Model file for the job. Use its own axes, mm. A direction names the side the tool comes from. Coordinates: 2 decimals unless noted, no trailing zeros. Loops run counter-clockwise (first coordinate to the right, second up) from the corner with the lowest first, then second, coordinate; pieces in that order, holes last. Notation, with made-up numbers: M -30.5,-29.5 L 8.5,-29.5 A16 ccw 8.5,-2.5 Z; hole C 43.5,59.25 d7. An arc over 180 degrees is marked long. One line per question, with ' | ' between items. Start each with the question number.
```python
from build123d import *

# Parameters (mm, degrees)
PAD_DEPTH       = 99.5
POCKET_DEPTH    = 106.001
POCKET001_DEPTH = 105
POCKET002_DEPTH = 37
POCKET003_DEPTH = 37
SKETCH005_W     = 30
SKETCH005_H     = 16.444138
POCKET004_DEPTH = 149


with BuildPart() as part:
    # Sketch → Pad (new body)
    with BuildSketch(Plane.XY):
        with BuildLine():
            Line((-53, 15), (-53, -29))
            ThreePointArc((-53, -29), (0, -82), (53, -29))
            Line((53, 15), (53, -29))
            ThreePointArc((53, 15), (48.606602, 25.606602), (38, 30))
            Line((-38, 30), (38, 30))
            ThreePointArc((-38, 30), (-48.606602, 25.606602), (-53, 15))
        make_face()
    extrude(amount=PAD_DEPTH)

    # Sketch001 (on DatumPlane) → Pocket (cut, through all)
    with BuildSketch(Plane.YZ.offset(53)):
        with BuildLine():
            ThreePointArc((30, 99.5), (-33.496233, 81.683249), (-82, 37))
            Line((-82, 37), (-89.555687, 37))
            Line((-89.555687, 106.401093), (-89.555687, 37))
            Line((30, 106.401093), (-89.555687, 106.401093))
            Line((30, 99.5), (30, 106.401093))
        make_face()
    extrude(amount=-POCKET_DEPTH, mode=Mode.SUBTRACT)

    # Sketch002 (on DatumPlane) → Pocket001 (cut)
    with BuildSketch(Plane.XY.offset(106)):
        with BuildLine():
            Line((-52, -29), (-16, -29))
            Line((-16, -29), (-16, -78.477268))
            ThreePointArc((-52, -29), (-42.047592, -59.594117), (-16, -78.477268))
        make_face()
        with BuildLine():
            Line((-15, 29), (15, 29))
            Line((15, 29), (15, -78.789557))
            ThreePointArc((-15, -78.789557), (0, -81), (15, -78.789557))
            Line((-15, 29), (-15, -78.789557))
        make_face()
        with BuildLine():
            Line((52, -29), (16, -29))
            Line((16, -29), (16, -78.477268))
            ThreePointArc((16, -78.477268), (42.047592, -59.594117), (52, -29))
        make_face()
        with BuildLine():
            Line((-16, 29), (-38.000001, 29))
            ThreePointArc((-38.000001, 29), (-47.850607, 24.850607), (-52, 15))
            Line((-52, 15), (-52, -28))
            Line((-52, -28), (-16, -28))
            Line((-16, -28), (-16, 29))
        make_face()
        with BuildLine():
            Line((16, 29), (38, 29))
            ThreePointArc((52, 15), (47.899495, 24.899495), (38, 29))
            Line((52, 15), (52, -28))
            Line((52, -28), (16, -28))
            Line((16, -28), (16, 29))
        make_face()
    extrude(amount=-POCKET001_DEPTH, mode=Mode.SUBTRACT)

    # Sketch003 (on DatumPlane) → Pocket002 (cut)
    with BuildSketch(Plane.YZ.offset(53)):
        Polygon((-29, 19), (-81, 19), (-81, 99.5), (-29.5, 99.5), (30, 99.5), (30, 82), (-29, 82), align=None)
    extrude(amount=-POCKET002_DEPTH, mode=Mode.SUBTRACT)

    # Sketch004 (on DatumPlane) → Pocket003 (cut)
    with BuildSketch(Plane(origin=(-53, 0, 0), x_dir=(0, -1, 0), z_dir=(-1, 0, 0))):
        Polygon((81, 38), (29, 38), (29, 68), (-30, 68), (-30, 99.5), (81, 99.5), align=None)
    extrude(amount=-POCKET003_DEPTH, mode=Mode.SUBTRACT)

    # Sketch005 (on DatumPlane) → Pocket004 (cut)
    with BuildSketch(Plane(origin=(-53, -120, 0), x_dir=(1, 0, 0), z_dir=(0, -1, 0))):
        with Locations((53, 46.222069)):
            Rectangle(SKETCH005_W, SKETCH005_H)
    extrude(amount=-POCKET004_DEPTH, mode=Mode.SUBTRACT)


solid = part.part
```
(1) Band-saw the part on D-D on z = 46. Write the cut outline in (x, y), then the cut area to 3 significant figures.
(2) 3-axis set-ups, long thin cutter, end or side, ignore diameter. For faces 1 (the face through (-52.4, -12.7, 68)), 2 (the face through (48.72, 25.49, 40.43)), 3 (the face through (35, -29, 42)), 4 (the face through (42.8, -59.8, 19)): which of +Z, -Z, +X, -X, +Y, -Y reach the whole face in a straight line?
(3) Pin check, flat tips, straight feed: P1, Ø5, axis at x = 8.5, z = 52.5, coming from the -Y side; P2, Ø11, axis at x = 26.5, y = -48.5, coming from the +Z side; P3, Ø11, axis at x = -40, y = -61.5, coming from the +Z side. Stop position of each tip, or through.
(4) Two-plate mould, pull along Y, no slides. Class faces 5 (the face through (15.482, -31.56, 82.744)), 6 (the face through (-47.7, 25, 35)), 7 (the face through (-1, 30, 38)), 8 (the face through (52.4, 11.6, 82)): pulls with the +Y half, pulls with the -Y half, needs draft (parallel to the pull), parting line crosses it, or undercut.
(5) Band-saw the part on C-C on y = 1.5. Write the cut outline in (x, z), then the cut area to 3 significant figures.
(6) Drill centre lines: line 1 (X direction, y = -18, z = 69); line 2 (X direction, y = 11.5, z = 60.5); line 3 (X direction, y = -41.5, z = 45.5). Where is each one in solid material? Low to high. Write a range as [from, to].
(7) Band-saw the part on B-B on x = 0. Write the cut outline in (y, z), then the cut area to 3 significant figures.
(8) Band-saw the part on A-A on z = 8.5. Write the cut outline in (x, y).
Computed values:
1) outline: M -53,-29 L -16,-29 L -16,-75.43 L -15,-75.43 L -15,29 L 15,29 L 15,-75.43 L 16,-75.43 L 16,-29 L 53,-29 L 53,15 A15 ccw 38,30 L -38,30 A15 ccw -53,15 Z; hole M -52,-28 L -16,-28 L -16,29 L -38,29 A14.17 ccw -52,15 Z; hole M 16,-28 L 52,-28 L 52,15 A14 ccw 38,29 L 16,29 Z | area: 491 mm^2
2) face 1: +Z, -X, +Y, -Y | face 2: +Z, -Z, +X, +Y | face 3: +Z | face 4: +Z, +X, -Y
3) P1: y = 29 | P2: z = 1 | P3: z = 38
4) face 5: pulls with the -Y half | face 6: undercut | face 7: pulls with the +Y half | face 8: needs draft
5) outline: M -53,0 L 53,0 L 53,82 L 52,82 L 52,1 L 16,1 L 16,95.48 L 15,95.48 L 15,1 L -15,1 L -15,95.48 L -16,95.48 L -16,1 L -52,1 L -52,68 L -53,68 Z | area: 443 mm^2
6) line 1: [-16, -15], [15, 16], [52, 53] | line 2: [-53, -52], [-16, -15], [15, 16], [52, 53] | line 3: [-16, -15], [15, 16]
7) outline: M -82,0 L 30,0 L 30,99.5 A141.36 ccw 29,99.46 L 29,1 L -81,1 L -81,38 L -81.32,38 A141.36 ccw -82,37 Z | area: 247 mm^2
8) outline: M -53,-29 A53 ccw 53,-29 L 53,15 A15 ccw 38,30 L -38,30 A15 ccw -53,15 Z; hole M -52,-29 A52 ccw -16,-78.48 L -16,-29 Z; hole M -52,-28 L -16,-28 L -16,29 L -38,29 A14.17 ccw -52,15 Z; hole M -15,-78.79 A52 ccw 15,-78.79 L 15,29 L -15,29 Z; hole M 16,-78.48 A52 ccw 52,-29 L 16,-29 Z; hole M 16,-28 L 52,-28 L 52,15 A14 ccw 38,29 L 16,29 Z
